CAD build for the part. Positions are in the model's coordinates, mm. Coordinates: 2 decimals unless noted, no trailing zeros. Order: outer loops, then holes, each group sorted by start corner. A loop starts at its lowest first (then second) coordinate and runs counter-clockwise, first axis right, second up. Notation, with made-up numbers: M 84,71.25 L 115,71.25 A30 ccw 115,109.25 Z; hole C -2.5,11.5 d9. An arc over 180 degrees is marked long. Write item = value, one per line.
from build123d import *

# Parameters (mm, degrees)
SKETCH2_W           = 110
SKETCH2_H           = 56.3
BOSS_EXTRUDE1_DEPTH = 12.7
HOLE_D              = 3.175
HOLE_DEPTH          = 31.75
HOLE_CSINK_D        = 10.16
HOLE_CSINK_ANGLE    = 82
HOLE_TIP            = 0.953866233
HOLE1_D             = 3.175
HOLE1_DEPTH         = 31.75
HOLE1_CSINK_D       = 10.16
HOLE1_CSINK_ANGLE   = 82
HOLE1_TIP           = 0.953866233


with BuildPart() as part:
    # Sketch2 → Boss-Extrude1 (new body)
    with BuildSketch(Plane.XY):
        with Locations((-286.304465963, 40.85)):
            Rectangle(SKETCH2_W, SKETCH2_H)
    extrude(amount=-BOSS_EXTRUDE1_DEPTH)

    # Hole
    with Locations(Plane(origin=(-124.004465969, 277.286738577, 0), x_dir=(-1, 0, 0), z_dir=(0, 0, 1))):
        with Locations((113.649999994, 236.436738577), (207.774999994, 236.436738577)):
            CounterSinkHole(HOLE_D / 2, HOLE_CSINK_D / 2, depth=HOLE_DEPTH, counter_sink_angle=HOLE_CSINK_ANGLE)
            with Locations((0, 0, -(HOLE_DEPTH + HOLE_TIP / 2))):  # 118° drill point
                Cone(0, HOLE_D / 2, HOLE_TIP, mode=Mode.SUBTRACT)

    # Hole1
    with Locations(Plane(origin=(-124.004465969, 88.05, -14.975709941), x_dir=(1, 0, 0), z_dir=(0, 1, 0))):
        with Locations((-162.299999994, -8.625709941), (-113.649999994, 50.157623392), (-113.649999994, 102.590956725), (162.299999994, -8.625709941), (113.649999994, 50.157623392), (113.649999994, 102.590956725), (63.85, 161.374290059), (0, 161.374290059), (-63.85, 161.374290059)):
            CounterSinkHole(HOLE1_D / 2, HOLE1_CSINK_D / 2, depth=HOLE1_DEPTH, counter_sink_angle=HOLE1_CSINK_ANGLE)
            with Locations((0, 0, -(HOLE1_DEPTH + HOLE1_TIP / 2))):  # 118° drill point
                Cone(0, HOLE1_D / 2, HOLE1_TIP, mode=Mode.SUBTRACT)


solid = part.part
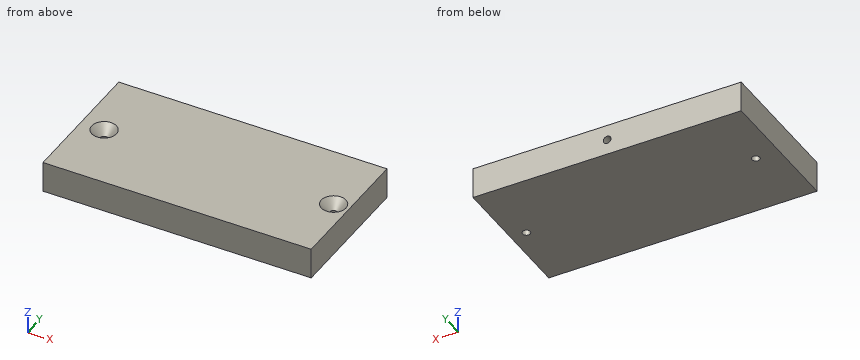
(1) Wall check: line 1 (X direction, y = 40.85, z = -6.5); line 2 (X direction, y = 60, z = -6.35); line 3 (X direction, y = 40, z = -6). Give the ranges that are in metal, low to high. Write a range as from..to.
Evaluation:
line_1 = -341.3..-333.37, -330.19..-239.24, -236.07..-231.3
line_2 = -341.3..-287.89, -284.72..-231.3
line_3 = -341.3..-333.12, -330.44..-239, -236.31..-231.3
(2) Pin check, flat tips, straight feed: pin 1 Ø5 at (x, y) = (-331.78, 40.85) entering from +Z; pin 2 Ø3.5 at (x, y) = (-237.65, 40.85) entering from +Z; pin 3 Ø8 at (x, y) = (-293, 47.5) entering from +Z. Stop position of each tip, or through.
Evaluation:
pin_1 = -2.97
pin_2 = -3.83
pin_3 = 0
(3) Slice it at A-A, the plane y = 40.85. Write the cut outline in (x, z).
Evaluation:
outline = M -341.3,-12.7 L -333.37,-12.7 L -333.37,-4.02 L -336.86,0 L -341.3,0 Z; M -330.19,-12.7 L -239.24,-12.7 L -239.24,-4.02 L -242.73,0 L -326.7,0 L -330.19,-4.02 Z; M -236.07,-12.7 L -231.3,-12.7 L -231.3,0 L -232.57,0 L -236.07,-4.02 Z
